```python
from build123d import *

# Parameters (mm, degrees)
SKETCH1_R           = 0.5
SKETCH1_R_2         = 6
SKETCH1_R_3         = 4
BOSS_EXTRUDE1_DEPTH = 12
SKETCH2_R           = 8.95
SKETCH2_R_2         = 9
CUT_EXTRUDE1_DEPTH  = 2
SKETCH3_R           = 0.5
CUT_EXTRUDE2_DEPTH  = 210.485083001
SKETCH4_R           = 3
CUT_EXTRUDE3_DEPTH  = 25
FILLET1_R           = 2


with BuildPart() as part:
    # Sketch1 → Boss-Extrude1 (new body)
    with BuildSketch(Plane(origin=(0, 0, 0), x_dir=(1, 0, 0), z_dir=(0, 1, 0))):
        with BuildLine():
            Line((55, 122), (55, 118))
            Line((55, 118), (0, 118))
            Line((0, 118), (0, 0))
            Line((0, 0), (30, 0))
            Line((30, 0), (30, 1))
            Line((30, 1), (72.5, 1))
            Line((72.5, 1), (72.5, -14))
            Line((72.5, -14), (82.5, -14))
            Line((82.5, -14), (82.5, 40))
            ThreePointArc((82.5, 40), (85, 93.984225439), (87.5, 40))
            Line((87.5, 40), (87.5, -14))
            Line((87.5, -14), (97.5, -14))
            Line((97.5, -14), (97.5, 1))
            Line((97.5, 1), (140, 1))
            Line((140, 1), (140, 0))
            Line((140, 0), (170, 0))
            Line((170, 0), (170, 118))
            Line((170, 118), (115, 118))
            Line((115, 118), (115, 122))
            Line((115, 122), (55, 122))
        make_face()
        with Locations(Location((65, 116, 0), (0, 0, 270))):
            Circle(SKETCH1_R, mode=Mode.SUBTRACT)
        with Locations(Location((105, 116, 0), (0, 0, 90))):
            Circle(SKETCH1_R, mode=Mode.SUBTRACT)
        with Locations(Location((45, 114, 0), (0, 0, 270))):
            Circle(SKETCH1_R, mode=Mode.SUBTRACT)
        with Locations(Location((15, 114, 0), (0, 0, 270))):
            Circle(SKETCH1_R, mode=Mode.SUBTRACT)
        with Locations(Location((155, 114, 0), (0, 0, 90))):
            Circle(SKETCH1_R, mode=Mode.SUBTRACT)
        with Locations(Location((125, 114, 0), (0, 0, 90))):
            Circle(SKETCH1_R, mode=Mode.SUBTRACT)
        with Locations(Location((15, 30, 0), (0, 0, 270))):
            Circle(SKETCH1_R_2, mode=Mode.SUBTRACT)
        with Locations(Location((155, 10, 0), (0, 0, 270))):
            Circle(SKETCH1_R_3, mode=Mode.SUBTRACT)
        with Locations(Location((15, 10, 0), (0, 0, 90))):
            Circle(SKETCH1_R_3, mode=Mode.SUBTRACT)
        with Locations(Location((85, 116, 0), (0, 0, 270))):
            Circle(SKETCH1_R, mode=Mode.SUBTRACT)
        with BuildLine():
            ThreePointArc((71.195976155, 101.316654464), (58.801693757, 93.132531682), (50.617570975, 80.738249284))
            ThreePointArc((50.617570975, 80.738249284), (52.561549872, 76.186222697), (57.113576458, 78.130201594))
            ThreePointArc((57.113576458, 78.130201594), (63.751441225, 88.182784214), (73.804023845, 94.820648981))
            ThreePointArc((73.804023845, 94.820648981), (75.748002742, 99.372675567), (71.195976155, 101.316654464))
        make_face(mode=Mode.SUBTRACT)
        with BuildLine():
            ThreePointArc((98.804023845, 101.316654464), (111.198306243, 93.132531682), (119.382429025, 80.738249284))
            ThreePointArc((119.382429025, 80.738249284), (117.438450128, 76.186222697), (112.886423542, 78.130201594))
            ThreePointArc((112.886423542, 78.130201594), (106.248558775, 88.182784214), (96.195976155, 94.820648981))
            ThreePointArc((96.195976155, 94.820648981), (94.251997258, 99.372675567), (98.804023845, 101.316654464))
        make_face(mode=Mode.SUBTRACT)
        with BuildLine():
            ThreePointArc((71.195976155, 32.551796414), (58.801693757, 40.735919196), (50.617570975, 53.130201594))
            ThreePointArc((50.617570975, 53.130201594), (52.561549872, 57.682228181), (57.113576458, 55.738249284))
            ThreePointArc((57.113576458, 55.738249284), (63.751441225, 45.685666664), (73.804023845, 39.047801898))
            ThreePointArc((73.804023845, 39.047801898), (75.748002742, 34.495775311), (71.195976155, 32.551796414))
        make_face(mode=Mode.SUBTRACT)
        with BuildLine():
            ThreePointArc((98.804023845, 32.551796414), (111.198306243, 40.735919196), (119.382429025, 53.130201594))
            ThreePointArc((119.382429025, 53.130201594), (117.438450128, 57.682228181), (112.886423542, 55.738249284))
            ThreePointArc((112.886423542, 55.738249284), (106.248558775, 45.685666664), (96.195976155, 39.047801898))
            ThreePointArc((96.195976155, 39.047801898), (94.251997258, 34.495775311), (98.804023845, 32.551796414))
        make_face(mode=Mode.SUBTRACT)
    extrude(amount=BOSS_EXTRUDE1_DEPTH)

    # Sketch2 → Cut-Extrude1 (cut)
    with BuildSketch(Plane(origin=(0, 12, 0), x_dir=(1, 0, 0), z_dir=(0, 1, 0))):
        with Locations(Location((31, 66.934225439, 0), (0, 0, 270))):
            Circle(SKETCH2_R)
        with Locations(Location((139.15, 66.934225439, 0), (0, 0, 270))):
            Circle(SKETCH2_R_2)
    extrude(amount=-CUT_EXTRUDE1_DEPTH, mode=Mode.SUBTRACT)

    # Sketch3 → Cut-Extrude2 (cut, through all)
    with BuildSketch(Plane(origin=(0, 10, 0), x_dir=(1, 0, 0), z_dir=(0, 1, 0))):
        with Locations(Location((31, 66.934225439, 0), (0, 0, 270))):
            Circle(SKETCH3_R)
        with Locations(Location((139.15, 66.934225439, 0), (0, 0, 270))):
            Circle(SKETCH3_R)
    extrude(amount=-CUT_EXTRUDE2_DEPTH, mode=Mode.SUBTRACT)

    # Sketch4 → Cut-Extrude3 (cut)
    with BuildSketch(Plane.ZY.offset(-72.5)):
        with Locations((6.5, 6)):
            Circle(SKETCH4_R)
    extrude(amount=-CUT_EXTRUDE3_DEPTH, mode=Mode.SUBTRACT)

    # Fillet1
    # the kernel refuses this fillet: 2 mm, written as the material it adds along each edge
    with BuildSketch(Plane(origin=(72.5, 0, -1), x_dir=(-1, 0, 0), z_dir=(0, 1, 0))) as fillet1_piece_1:
        with BuildLine():
            CenterArc((FILLET1_R, FILLET1_R), FILLET1_R, 180, 90)
            Line((0, FILLET1_R), (0, 0))
            Line((0, 0), (FILLET1_R, 0))
        make_face()
    extrude(amount=12)
    with BuildSketch(Plane(origin=(97.5, 0, -1), x_dir=(1, 0, 0), z_dir=(0, 1, 0))) as fillet1_piece_2:
        with BuildLine():
            CenterArc((FILLET1_R, -FILLET1_R), FILLET1_R, 90, 90)
            Line((0, -FILLET1_R), (0, 0))
            Line((0, 0), (FILLET1_R, 0))
        make_face()
    extrude(amount=12)
    # the kernel refuses this fillet: 2 mm, written as the material it takes off along each edge
    with BuildSketch(Plane(origin=(170, -5, 0), x_dir=(0, 0, -1), z_dir=(0, 1, 0)), Plane(origin=(97.5, -5, 14), x_dir=(0, 0, -1), z_dir=(0, 1, 0))) as fillet1_2_piece_1:
        with BuildLine():
            CenterArc((FILLET1_R, FILLET1_R), FILLET1_R, 180, 90)
            Line((0, FILLET1_R), (0, 0))
            Line((0, 0), (FILLET1_R, 0))
        make_face()
    extrude(amount=22, mode=Mode.SUBTRACT)
    with BuildSketch(Plane(origin=(140, -4.330127019, 0), x_dir=(1, 0, 0), z_dir=(0, 1, 0))) as fillet1_2_piece_2:
        with BuildLine():
            CenterArc((1.732050808, 2), FILLET1_R, 210, 60)
            Line((0, 1), (0, 0))
            Line((0, 0), (1.732050808, 0))
        make_face()
    extrude(amount=20.660254038, mode=Mode.SUBTRACT)
    with BuildSketch(Plane(origin=(72.5, -5, 14), x_dir=(0, 0, -1), z_dir=(0, 1, 0)), Plane(origin=(0, -5, 0), x_dir=(0, 0, -1), z_dir=(0, 1, 0))) as fillet1_2_piece_3:
        with BuildLine():
            CenterArc((FILLET1_R, -FILLET1_R), FILLET1_R, 90, 90)
            Line((0, -FILLET1_R), (0, 0))
            Line((0, 0), (FILLET1_R, 0))
        make_face()
    extrude(amount=22, mode=Mode.SUBTRACT)
    with BuildSketch(Plane(origin=(30, -4.330127019, 0), x_dir=(-1, 0, 0), z_dir=(0, 1, 0))) as fillet1_2_piece_4:
        with BuildLine():
            CenterArc((1.732050808, -2), FILLET1_R, 90, 60)
            Line((0, -1), (0, 0))
            Line((0, 0), (1.732050808, 0))
        make_face()
    extrude(amount=20.660254038, mode=Mode.SUBTRACT)


solid = part.part
```
CAD build for the part. Positions are in the model's coordinates, mm. A direction names the side the tool comes from. Give positions to 0.01 mm unless a question says otherwise; leave off trailing zeros. Write each loop counter-clockwise with the first axis right and the second up, starting at its lowest first coordinate (ties: lowest second). Pieces come first, ordered by that corner, then holes. Notation, with made-up numbers: M 29,-37.75 L 62,-37.75 A15 ccw 62,-17.75 Z; hole C 7.5,54.5 d6. An arc over 180 degrees is marked long. Return JSON: item names as keys, results as strings. Group by question number.
(1) Band-saw the part on D-D (z = -61.5). Give the cut face in (x, y).
(2) Band-saw the part on C-C (x = 35.5). Give the cut face in (y, z).
(3) 3-axis set-ups, long thin cutter, end or side, ignore diameter. For faces 5 (the face through (119, 6, -1)), 6 (the face through (148.073, 11.014, -68.106)), 7 (the face through (97.5, 3, 8)), 8 (the face through (63.63, 5.92, -88.06)): which of +Z, -Z, +X, -X, +Y, -Y reach the whole face in a straight line?
(4) Band-saw the part on B-B (z = -16). Give the cut face in (x, y).
(5) Mould opens along X. For faces 1 (the face through (117.51, 5.916, -76.216)), 2 (the face through (58.95, 5.92, -93.28)), 3 (the face through (155, 6, 0)), 4 (the face through (55, 6, -120)) say: pulls with the +X half, pulls with the -X half, needs draft (parallel to the pull), parting line crosses it, or undercut.
(6) Flat gauge pins, fed straight in: pin 1 Ø6 at (x, y) = (49.5, 8.5) entering from +Z; pin 2 Ø1.2 at (y, z) = (4, -120) entering from -X; pin 3 Ø3 at (y, z) = (4.5, -120) entering from +X. Where does each tip first touch, or does it go through?
(7) Band-saw the part on A-A (z = -30). Give the cut face in (x, y).
(8) Drill centre lines: L1, parallel to X at y = 4.75, z = -114; L2, parallel to X at y = 6.25, z = -116; L3, parallel to X at y = 11, z = 8. Where is each one in solid material? Low to high. Write a range as [from, to].
Entries:
{
 "1": {"outline": "M 0,0 L 58.5,0 L 58.5,12 L 38.11,12 L 38.11,10 L 23.89,10 L 23.89,12 L 0,12 Z; M 111.5,0 L 170,0 L 170,12 L 146.32,12 L 146.32,10 L 131.98,10 L 131.98,12 L 111.5,12 Z"},
 "2": {"outline": "M 0,-118 L 12,-118 L 12,-74.67 L 10,-74.67 L 10,-59.2 L 12,-59.2 L 12,-1 L 0,-1 Z"},
 "3": {"face 5": "+Z, +Y, -Y", "face 6": "+Y", "face 7": "+Z, +X, +Y, -Y", "face 8": "+Y, -Y"},
 "4": {"outline": "M 0,0 L 82.5,0 L 82.5,12 L 0,12 Z; M 87.5,0 L 170,0 L 170,12 L 87.5,12 Z"},
 "5": {"face 1": "undercut", "face 2": "undercut", "face 3": "needs draft", "face 4": "pulls with the -X half"},
 "6": {"pin 1": "stops at z = -1", "pin 2": "stops at x = 55", "pin 3": "stops at x = 115"},
 "7": {"outline": "M 0,0 L 9,0 L 9,12 L 0,12 Z; M 21,0 L 82.5,0 L 82.5,12 L 21,12 Z; M 87.5,0 L 170,0 L 170,12 L 87.5,12 Z"},
 "8": {"L1": "x = [0, 14.5], [15.5, 44.5], [45.5, 124.5], [125.5, 154.5], [155.5, 170]", "L2": "x = [0, 64.5], [65.5, 84.5], [85.5, 104.5], [105.5, 170]", "L3": "x = [72.5, 82.5], [87.5, 97.5]"}
}
